Design review of the part built by this model. Coordinates are the model's own, in mm. Face numbers are marked on the shaded views. A direction names the side the tool comes from. Round coordinates to 2 decimals unless told otherwise and drop trailing zeros. Loops run counter-clockwise (first coordinate to the right, second up) from the corner with the lowest first, then second, coordinate; pieces in that order, holes last. Notation, with made-up numbers: M 31.25,-0.5 L 71.25,-0.5 A14 ccw 71.25,17.5 Z; hole C -24.75,-33.5 d8. An arc over 180 degrees is marked long. One line per item, written item: value. Start each with the question number.
Item 1: We need section A-A (y = 5.75). Write out the cut boundary in (x, z), then the cut area to 3 significant figures.
Item 2: For the marked faces 1, 2 and 3, list the 3-axis set-ups (+Z, -Z, +X, -X, +Y, -Y) from which the entire face can be reached by the end or side of a thin tool; tool diameter is ignored.
Item 3: We need section C-C (x = 19). Write out the cut boundary in (y, z), then the cut area to 3 significant figures.
Item 4: We need section B-B (z = 1.7). Write out the cut boundary in (x, y).
Item 5: Clearance check with flat-ended pins moving along their axes: pin 1 (1 mm diameter, centred on x = 10.5, y = 1.5, fed in from -Z); pin 2 (2.5 mm diameter, centred on x = 0, z = 3, fed in from +Y). State where each tip first meets the part, or that it passes through.
Item 6: For line 1 along Y through (x, z) = (16, 1.55); line 2 along Y through (x, z) = (0, 1.2); line 3 along X through (y, z) = (8.25, 4), list the stretches that pass through material, from the lowest coordinate up.
Item 7: We need section D-D (x = 32). Write out the cut boundary in (y, z).
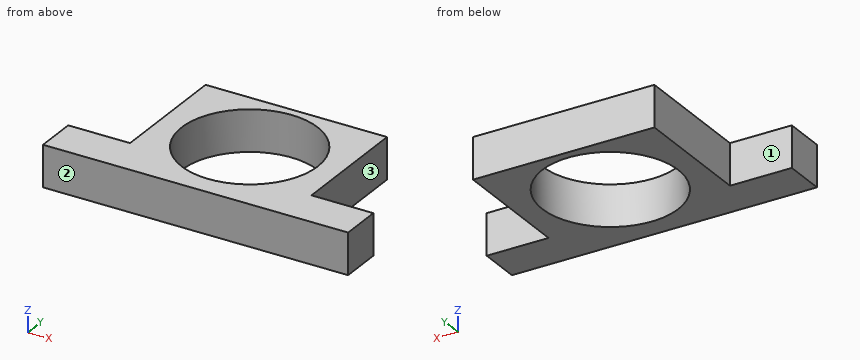
from build123d import *

# Parameters (mm, degrees)
F0_W     = 37
F0_H     = 5
F1_DEPTH = 5
F2_W     = 22
F2_H     = 5
F3_DEPTH = 15
F4_R     = 8.25
F5_DEPTH = 25.4


with BuildPart() as f1:
    # F0 (on Top) → F1 (new body)
    with BuildSketch(Plane.XY):
        with Locations((16.031665, -2.5)):
            Rectangle(F0_W, F0_H)
    extrude(amount=F1_DEPTH)

    # F2 (on face) → F3 (join)
    with BuildSketch(Plane(origin=(0, 0, 0), x_dir=(-1, 0, 0), z_dir=(0, 1, 0))):
        with Locations((-16.031665, 2.5)):
            Rectangle(F2_W, F2_H)
    extrude(amount=F3_DEPTH)

    # F4 (on face) → F5 (cut)
    with BuildSketch(Plane.XY.offset(5)):
        with Locations((16.031665, 5.75)):
            Circle(F4_R)
    extrude(amount=-F5_DEPTH, mode=Mode.SUBTRACT)


solid = f1.part
A:
1. outline: M 5.03,0 L 7.78,0 L 7.78,5 L 5.03,5 Z; M 24.28,0 L 27.03,0 L 27.03,5 L 24.28,5 Z
1. area: 27.5 mm2
2. face 1: +Z, -Z, -X, +Y
2. face 2: +Z, -Z, +X, -X, -Y
2. face 3: +Z, -Z, +X, +Y
3. outline: M -5,0 L -1.95,0 L -1.95,5 L -5,5 Z; M 13.45,0 L 15,0 L 15,5 L 13.45,5 Z
3. area: 23.0 mm2
4. outline: M -2.47,-5 L 34.53,-5 L 34.53,0 L 27.03,0 L 27.03,15 L 5.03,15 L 5.03,0 L -2.47,0 Z; hole C 16.03,5.75 d16.5
5. pin 1: through
5. pin 2: y = 0
6. line 1: -5 to -2.5, 14 to 15
6. line 2: -5 to 0
6. line 3: 5.03 to 8.17, 23.89 to 27.03
7. outline: M -5,0 L 0,0 L 0,5 L -5,5 Z
